The drawing under review shows one solid part. Ordinate dimensions are in mm from its lowest x, y, z. Round coordinates to 2 decimals unless told otherwise and drop trailing zeros. Write each loop counter-clockwise with the first axis right and the second up, starting at its lowest first coordinate (ties: lowest second). Pieces come first, ordered by that corner, then holes.
Item 1: Add section A-A (y = 1.1). Give the boundary of the cut face in (x, z), plus the area to 3 significant figures.
Item 2: Clearance check with flat-ended pins moving along their axes: pin 1 Ø0.9 at (x, y) = (21.5, 1) entering from +Z; pin 2 Ø0.9 at (x, y) = (22, 0.5) entering from -Z; pin 3 Ø0.8 at (y, z) = (1, 36) entering from +X. State where each tip first meets the part, or that it passes through.
Item 3: Add section D-D (z = 39). Give the boundary of the cut face in (x, y).
Item 4: Add section C-C (z = 20.95). Give the boundary of the cut face in (x, y), plus the area to 3 significant figures.
Item 5: Add section B-B (x = 20.95). Give the boundary of the cut face in (y, z), plus the area to 3 significant figures.
Item 6: To check wall thickness, follow L1, parallel to Y at x = 28.5, z = 10; L2, parallel to X at y = 1.45, z = 35.5; L3, parallel to X at y = 2.65, z = 27.5. State the ranges of each line that lie inside material, in increasing order.
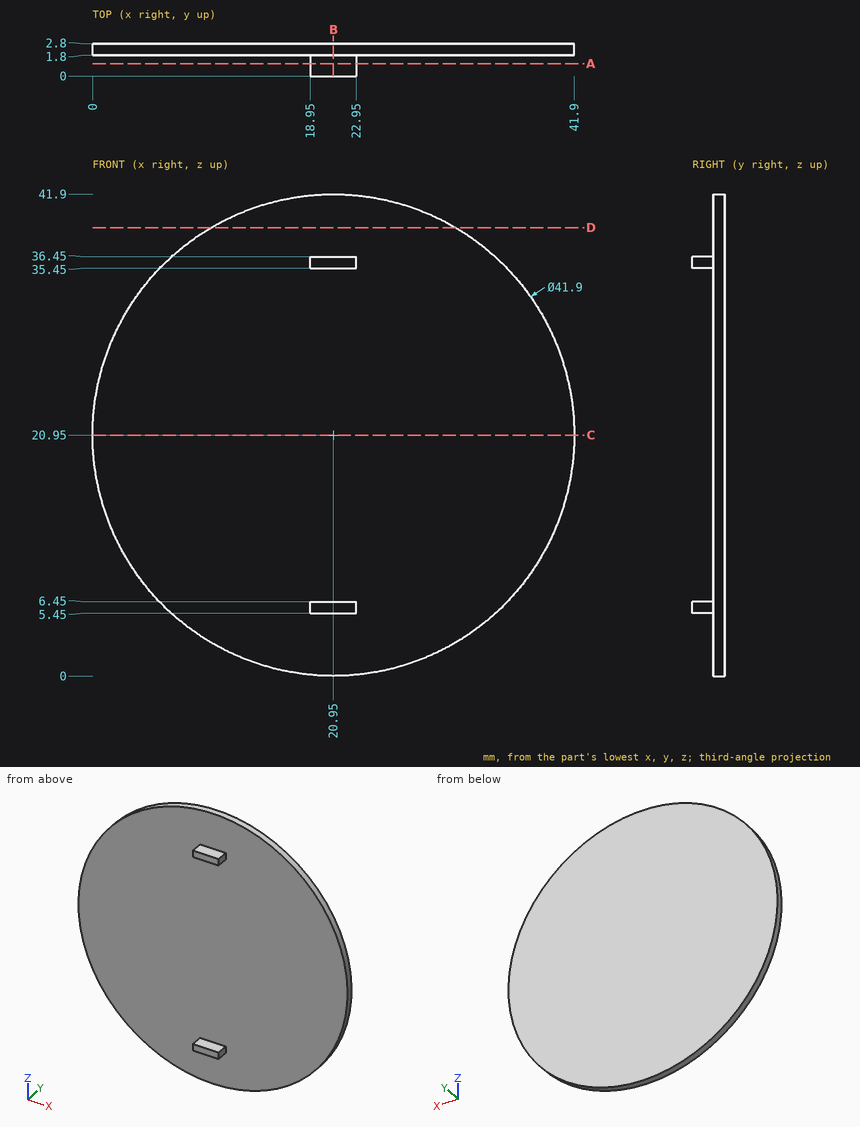
Numbers:
1. outline: (18.95, 5.45) - (22.95, 5.45) - (22.95, 6.45) - (18.95, 6.45) - close; (18.95, 35.45) - (22.95, 35.45) - (22.95, 36.45) - (18.95, 36.45) - close
1. area: 8.00 mm2
2. pin 1: stops at z = 36.45
2. pin 2: stops at z = 5.45
2. pin 3: stops at x = 22.95
3. outline: (10.32, 1.8) - (31.58, 1.8) - (31.58, 2.8) - (10.32, 2.8) - close
4. outline: (0, 1.8) - (41.9, 1.8) - (41.9, 2.8) - (0, 2.8) - close
4. area: 41.9 mm2
5. outline: (0, 5.45) - (1.8, 5.45) - (1.8, 0) - (2.8, 0) - (2.8, 41.9) - (1.8, 41.9) - (1.8, 36.45) - (0, 36.45) - (0, 35.45) - (1.8, 35.45) - (1.8, 6.45) - (0, 6.45) - close
5. area: 45.5 mm2
6. L1: y = 1.8 to 2.8
6. L2: x = 18.95 to 22.95
6. L3: x = 1.05 to 40.85
